```python
from build123d import *

# Parameters (mm, degrees)
PAD_DEPTH       = 18
POCKET_DEPTH    = 16
POCKET001_DEPTH = 5
POCKET002_DEPTH = 5
POCKET003_DEPTH = 4


with BuildPart() as part:
    # Sketch → Pad (new body)
    with BuildSketch(Plane.XY):
        with BuildLine():
            Line((-13.75, -16.5), (13.75, -16.5))
            ThreePointArc((13.75, -16.5), (18.699747, -14.449747), (20.75, -9.5))
            Line((20.75, -9.5), (20.75, 9.5))
            ThreePointArc((20.75, 9.5), (18.699747, 14.449747), (13.75, 16.5))
            Line((13.75, 16.5), (-13.75, 16.5))
            ThreePointArc((-13.75, 16.5), (-18.699747, 14.449747), (-20.75, 9.5))
            Line((-20.75, 9.5), (-20.75, -9.5))
            ThreePointArc((-20.75, -9.5), (-18.699747, -14.449747), (-13.75, -16.5))
        make_face()
    extrude(amount=PAD_DEPTH)

    # Sketch001 (on Face10 of Pad) → Pocket (cut)
    with BuildSketch(Plane.XY.offset(18)):
        with BuildLine():
            Line((-19.25, 11.5), (-19.25, -11.5))
            ThreePointArc((-19.25, -11.5), (-18.078427, -14.328427), (-15.25, -15.5))
            Line((-15.25, -15.5), (15.25, -15.5))
            ThreePointArc((15.25, -15.5), (18.078427, -14.328427), (19.25, -11.5))
            Line((19.25, -11.5), (19.25, 11.5))
            ThreePointArc((19.25, 11.5), (18.078427, 14.328427), (15.25, 15.5))
            Line((15.25, 15.5), (-15.25, 15.5))
            ThreePointArc((-15.25, 15.5), (-18.078427, 14.328427), (-19.25, 11.5))
        make_face()
    extrude(amount=-POCKET_DEPTH, mode=Mode.SUBTRACT)

    # Sketch002 (on Face1 of Pocket) → Pocket001 (cut)
    with BuildSketch(Plane.XZ.offset(16.5)):
        with BuildLine():
            Line((-6, 18), (-6, 13))
            ThreePointArc((-6, 13), (-5.414214, 11.585786), (-4, 11))
            Line((-4, 11), (2, 11))
            ThreePointArc((2, 11), (3.414214, 11.585786), (4, 13))
            Line((4, 13), (4, 18))
            ThreePointArc((4, 18), (3.414214, 19.414214), (2, 20))
            Line((2, 20), (-4, 20))
            ThreePointArc((-4, 20), (-5.414214, 19.414214), (-6, 18))
        make_face()
    extrude(amount=-POCKET001_DEPTH, mode=Mode.SUBTRACT)

    # Sketch003 (on Face13 of Pocket001) → Pocket002 (cut)
    with BuildSketch(Plane(origin=(0, 16.5, 0), x_dir=(-1, 0, 0), z_dir=(0, 1, 0))):
        with BuildLine():
            Line((-12, 18), (-12, 12))
            ThreePointArc((-12, 12), (-11.414214, 10.585786), (-10, 10))
            Line((-10, 10), (10, 10))
            ThreePointArc((10, 10), (11.414214, 10.585786), (12, 12))
            Line((12, 12), (12, 18))
            ThreePointArc((12, 18), (11.414214, 19.414214), (10, 20))
            Line((10, 20), (-10, 20))
            ThreePointArc((-10, 20), (-11.414214, 19.414214), (-12, 18))
        make_face()
    extrude(amount=-POCKET002_DEPTH, mode=Mode.SUBTRACT)

    # Sketch004 (on Face4 of Pocket002) → Pocket003 (cut)
    with BuildSketch(Plane.XY.offset(18)):
        with BuildLine():
            Line((15.2, 9), (15.2, -10))
            ThreePointArc((15.2, -10), (15.63934, -11.06066), (16.7, -11.5))
            Line((16.7, -11.5), (18.7, -11.5))
            ThreePointArc((18.7, -11.5), (19.76066, -11.06066), (20.2, -10))
            Line((20.2, -10), (20.2, 9))
            ThreePointArc((20.2, 9), (19.76066, 10.06066), (18.7, 10.5))
            Line((18.7, 10.5), (16.7, 10.5))
            ThreePointArc((16.7, 10.5), (15.63934, 10.06066), (15.2, 9))
        make_face()
    extrude(amount=-POCKET003_DEPTH, mode=Mode.SUBTRACT)


solid = part.part
```
Work out the finished part from the listing and answer in its coordinate system (mm). A direction names the side the tool comes from. Coordinates: 2 decimals unless noted, no trailing zeros. Loops run counter-clockwise (first coordinate to the right, second up) from the corner with the lowest first, then second, coordinate; pieces in that order, holes last. Notation, with made-up numbers: M -36.5,40 L -20.5,40 A14 cw -20.5,50 Z; hole C 16,4 d4. An arc over 180 degrees is marked long. Use CSV: the item, a comma, the result in double quotes. Start each with the question number.
(1) Consider line 1 (Y direction, x = -3, z = 3); line 2 (X direction, y = -9.5, z = 15.25); line 3 (X direction, y = 3, z = 3.5). Determine where each line is inside the solid, lowest interval first.
(2) Find section C-C, the plane y = -1. Give the vertices of the cut face in (x, z).
(3) For faces 1 (the face through (19.95, 9.83, 16.03)), 2 (the face through (12, 16, 15)), 3 (the face through (3.4, -16.01, 11.57)), determine the directions among +Z, -Z, +X, -X, +Y, -Y from which every point of the face is accessible in a straight line to the end or side of a thin tool.
(4) Find section D-D, the plane z = 12.5. Give the vertices of the cut face in (x, y).
(5) Given pin 1 Ø1.5 at (x, y) = (-14.5, -8.5) entering from +Z; pin 2 Ø0.5 at (y, z) = (16, 14) entering from -X; pin 3 Ø3 at (x, z) = (-16, 2) entering from -Y, each flat-ended and moving along its own axis, determine where each tip first touches the part or whether it passes through.
(6) Find section A-A, the plane z = 4.75. Give the vertices of the cut face in (x, y), then the cut area to 3 significant figures.
(7) Find section B-B, the plane x = 0.5. Give the vertices of the cut face in (y, z), then the cut area to 3 significant figures.
(8) For a pull along X with two mould halves and no side action, classify faces 4 (the face through (0, 15.5, 7)), 5 (the face through (0, 0, 0)), 6 (the face through (-18.75, -14.4, 8.87)) as +X half, -X half, draft (parallel to the pull), parting line (faces both ways), or undercut.
Recorded:
1,line 1,"y = -16.5 to -15.5, 15.5 to 16.5"
1,line 2,"x = -20.75 to -19.25, 20.2 to 20.75"
1,line 3,"x = -20.75 to -19.25, 19.25 to 20.75"
2,outline,"M -20.75,0 L 20.75,0 L 20.75,18 L 20.2,18 L 20.2,14 L 19.25,14 L 19.25,2 L -19.25,2 L -19.25,18 L -20.75,18 Z"
3,face 1,"+Z"
3,face 2,"+Z, +Y"
3,face 3,"+Z, +Y, -Y"
4,outline,"M -20.75,-9.5 A7 ccw -13.75,-16.5 L -5.94,-16.5 L -5.94,-15.5 L -15.25,-15.5 A4 cw -19.25,-11.5 L -19.25,11.5 A4 cw -15.25,15.5 L -12,15.5 L -12,16.5 L -13.75,16.5 A7 ccw -20.75,9.5 Z; M 3.94,-16.5 L 13.75,-16.5 A7 ccw 20.75,-9.5 L 20.75,9.5 A7 ccw 13.75,16.5 L 12,16.5 L 12,15.5 L 15.25,15.5 A4 cw 19.25,11.5 L 19.25,-11.5 A4 cw 15.25,-15.5 L 3.94,-15.5 Z"
5,pin 1,"stops at z = 2"
5,pin 2,"stops at x = -16.9"
5,pin 3,"stops at y = -16.46"
6,outline,"M -20.75,-9.5 A7 ccw -13.75,-16.5 L 13.75,-16.5 A7 ccw 20.75,-9.5 L 20.75,9.5 A7 ccw 13.75,16.5 L -13.75,16.5 A7 ccw -20.75,9.5 Z; hole M -19.25,-11.5 A4 ccw -15.25,-15.5 L 15.25,-15.5 A4 ccw 19.25,-11.5 L 19.25,11.5 A4 ccw 15.25,15.5 L -15.25,15.5 A4 ccw -19.25,11.5 Z"
6,area,"148 mm^2"
7,outline,"M -16.5,0 L 16.5,0 L 16.5,10 L 15.5,10 L 15.5,2 L -15.5,2 L -15.5,11 L -16.5,11 Z"
7,area,"83.0 mm^2"
8,face 4,"undercut"
8,face 5,"draft"
8,face 6,"-X half"
